from build123d import *

# Parameters (mm, degrees)
SKETCH2_R           = 2.5
SKETCH3_R           = 3.5
BOSS_EXTRUDE1_DEPTH = 15


with BuildPart() as part:
    # Sweep1: sweep along a path in Sketch1
    with BuildLine(Plane(origin=(0, 0, 0), x_dir=(0, 0, -1), z_dir=(1, 0, 0))) as sweep1_path:
        Line((0, 0), (0, 30))
        Line((0, 30), (-224.277396019, 91.890417139))
        Line((-224.277396019, 91.890417139), (-233, 87))
    # Sketch2 → Sweep1 (sweep)
    with BuildSketch(Plane(origin=(0, 87, 233), x_dir=(1, 0, 0), z_dir=(0, -0.489041714, 0.872260398))):
        Circle(SKETCH2_R)
    sweep(path=sweep1_path.line, transition=Transition.RIGHT)

    # Sketch3 → Boss-Extrude1 (add)
    with BuildSketch(Plane.XZ):
        Circle(SKETCH3_R)
    extrude(amount=-BOSS_EXTRUDE1_DEPTH)


solid = part.part
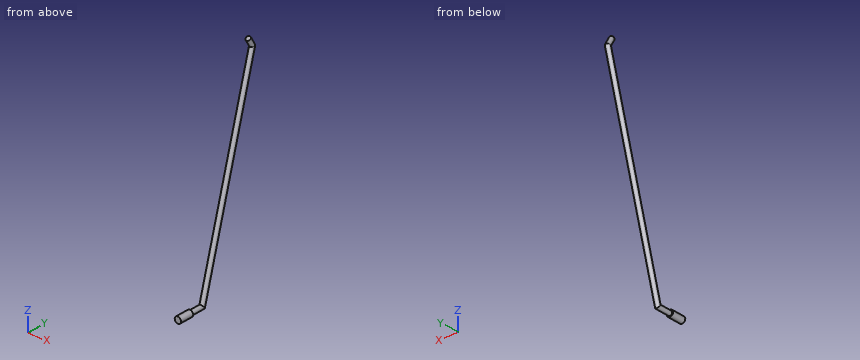
Model file for the job. Use its own axes, mm. Round coordinates to 2 decimals unless told otherwise and drop trailing zeros. Order: outer loops, then holes, each group sorted by start corner. A loop starts at its lowest first (then second) coordinate and runs counter-clockwise, first axis right, second up. Notation, with made-up numbers: M 44,-32.75 L 56,-32.75 A19 cw 56,-14.75 Z; hole C -19.5,-6 d3. An arc over 180 degrees is marked long. Write each question's results on one line, items separated by ' | '. Start each with the question number.
(1) Saw through at A-A, the plane x = 0. Give the cut face in (y, z), then the cut area to 3 significant figures.
(2) Drop flat-ended pins along their axis: pin 1 (10 mm diameter, centred on y = 66, z = 154, fed in from -X); pin 2 (2 mm diameter, centred on x = 1.5, z = -1.5, fed in from +Y); pin 3 (2 mm diameter, centred on x = -1, z = 54, fed in from +Y). Give the stop position or say it passes through.
(3) Probe probe 1 along X at (y, z) = (34, 14); probe 2 along Z at (x, y) = (-2.75, 11); probe 3 along Y at (x, z) = (1, 125.5). List the from-to ranges inside material, lowest first. Write a range as from..to.
Established:
1) outline: M 0,-3.5 L 15,-3.5 L 15,-2.5 L 31.9,-2.5 L 94.57,224.6 L 89.18,234.22 L 84.82,231.78 L 89.21,223.95 L 28.1,2.5 L 15,2.5 L 15,3.5 L 0,3.5 Z | area: 1,390 mm^2
2) pin 1: stops at x = -2.16 | pin 2: stops at y = 32.24 | pin 3: stops at y = 47.68
3) probe 1: x = -2.5..2.5 | probe 2: z = -2.17..2.17 | probe 3: y = 62.26..67.01
